Geometry check sheet. Reference: the model listing, model coordinates, mm. Face numbers are marked on the shaded views. A direction names the side the tool comes from. Coordinates: 2 decimals unless noted, no trailing zeros. Write each loop counter-clockwise with the first axis right and the second up, starting at its lowest first coordinate (ties: lowest second). Pieces come first, ordered by that corner, then holes. Notation, with made-up numbers: (88, -6) -> (139, -6) arc R19 cw to (139, 24) -> close; hole circle Ø9 at (18, -39.75). An arc over 180 degrees is marked (long way). Answer in a Markdown table with one row per item. Add a question column.
1. Cross-section at A-A on x = 19. Record the cut outline in (y, z), and give its area (3 significant figures).
2. Set-up check for the marked faces 4, 5, 6 and 7: record each of +Z, -Z, +X, -X, +Y, -Y from which the full face is reachable in a straight line by a thin tool's end or side.
3. Depth check by flat-ended pin: P1, Ø1.8, axis at x = 2, z = 2, coming from the -Y side; P2, Ø11.5, axis at x = 26, z = 24, coming from the +Y side; P3, Ø6, axis at y = 28, z = 21, coming from the -X side; P4, Ø1, axis at x = 25, y = 30, coming from the -Z side. Enter the tip coordinate at first touch or a pass-through.
4. Scan lines: L1, parallel to X at y = 1, z = 2; L2, parallel to Y at x = 3, z = 13.5; L3, parallel to Y at x = 22, z = 20.5. Record each from-to range of solid material in increasing order. Write a range as from..to.
5. Cross-section at B-B on z = 36. Record the cut outline in (x, y), and give its area (3 significant figures).
6. Cross-section at C-C on y = -1. Record the cut outline in (x, z), and give its area (3 significant figures).
7. Cross-section at D-D on z = 19. Record the cut outline in (x, y).
8. Mould release check, pull along Z, two halves, no side actions. Record for the marked faces 1, 2 and 3: pulls with the +Z half, pulls with the -Z half, needs draft (parallel to the pull), parting line crosses it, or undercut.
```python
from build123d import *

# Parameters (mm, degrees)
SKETCH_1_W      = 38
SKETCH_1_H      = 38
SKETCH_1_R      = 1
EXTRUDE_1_DEPTH = 1.5
SKETCH_2_R      = 0.636700884
SKETCH_2_R_2    = 0.447912605
SKETCH_2_R_3    = 0.577059181
SKETCH_2_R_4    = 0.454786346
EXTRUDE_2_DEPTH = 12
SKETCH_3_W      = 38
SKETCH_3_H      = 38
EXTRUDE_3_DEPTH = 1.5
SKETCH_4_R      = 7
EXTRUDE_4_DEPTH = 24
SKETCH_5_W      = 23.785325885
SKETCH_5_H      = 24.83133448
SKETCH_5_W_2    = 7.276581533
SKETCH_5_H_2    = 1.922772716
EXTRUDE_5_DEPTH = 6.6


with BuildPart() as part:
    # 草图1 → 凸台-拉伸1 (new body)
    with BuildSketch(Plane(origin=(0, 0, 0), x_dir=(1, 0, 0), z_dir=(0, 1, 0))):
        with Locations((19, -19)):
            Rectangle(SKETCH_1_W, SKETCH_1_H)
        with Locations(Location((2, -2, 0), (0, 0, 270))):
            Circle(SKETCH_1_R, mode=Mode.SUBTRACT)
        with Locations(Location((36, -2, 0), (0, 0, 270))):
            Circle(SKETCH_1_R, mode=Mode.SUBTRACT)
        with Locations(Location((36, -36, 0), (0, 0, 270))):
            Circle(SKETCH_1_R, mode=Mode.SUBTRACT)
        with Locations(Location((2, -36, 0), (0, 0, 270))):
            Circle(SKETCH_1_R, mode=Mode.SUBTRACT)
    extrude(amount=EXTRUDE_1_DEPTH)

    # 草图2 → 凸台-拉伸2 (add)
    with BuildSketch(Plane(origin=(0, 1.5, 0), x_dir=(1, 0, 0), z_dir=(0, 1, 0))):
        with Locations(Location((4.128486493, -34.030688728, 0), (0, 0, 270))):
            Circle(SKETCH_2_R)
        with Locations(Location((4.765187377, -3.05973858, 0), (0, 0, 270))):
            Circle(SKETCH_2_R_2)
        with Locations(Location((32.780026277, -2.611825975, 0), (0, 0, 270))):
            Circle(SKETCH_2_R_3)
        with Locations(Location((33.644120334, -34.030688728, 0), (0, 0, 270))):
            Circle(SKETCH_2_R_4)
    extrude(amount=EXTRUDE_2_DEPTH)

    # 草图3 → 凸台-拉伸3 (add)
    with BuildSketch(Plane(origin=(0, 13.5, 0), x_dir=(1, 0, 0), z_dir=(0, 1, 0))):
        with Locations((19, -19)):
            Rectangle(SKETCH_3_W, SKETCH_3_H)
    extrude(amount=EXTRUDE_3_DEPTH)

    # 草图4 → 凸台-拉伸4 (add)
    with BuildSketch(Plane(origin=(0, 15, 0), x_dir=(1, 0, 0), z_dir=(0, 1, 0))):
        with Locations(Location((19, -19, 0), (0, 0, 270))):
            Circle(SKETCH_4_R)
    extrude(amount=EXTRUDE_4_DEPTH)

    # 草图5 → 凸台-拉伸5 (add)
    with BuildSketch(Plane(origin=(0, 0, 0), x_dir=(-1, 0, 0), z_dir=(0, -1, 0))):
        with Locations((-19.113696587, -19.568482932)):
            Rectangle(SKETCH_5_W, SKETCH_5_H)
        with Locations((-18.818085462, -0.961386358)):
            Rectangle(SKETCH_5_W_2, SKETCH_5_H_2)
    extrude(amount=EXTRUDE_5_DEPTH)


solid = part.part
```
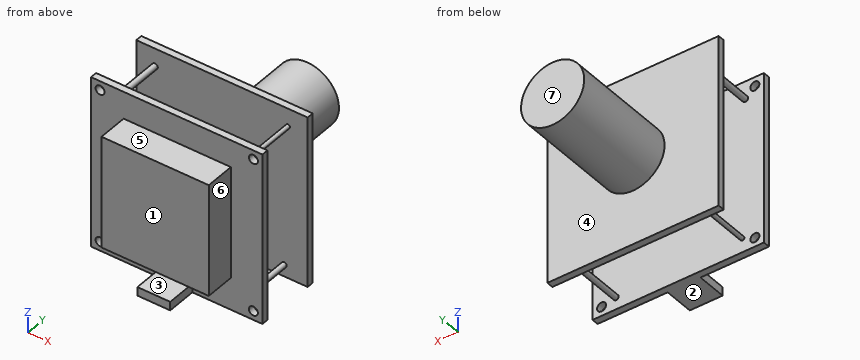
Results found:
| question | item | result |
|---|---|---|
| 1 | outline | (-6.6, 0) -> (1.5, 0) -> (1.5, 38) -> (0, 38) -> (0, 31.98) -> (-6.6, 31.98) -> (-6.6, 7.15) -> (0, 7.15) -> (0, 1.92) -> (-6.6, 1.92) -> close; (13.5, 0) -> (15, 0) -> (15, 12) -> (39, 12) -> (39, 26) -> (15, 26) -> (15, 38) -> (13.5, 38) -> close |
| 1 | area | 627 mm^2 |
| 2 | face 4 | +Y |
| 2 | face 5 | +Z, +X, -X, -Y |
| 2 | face 6 | +Z, -Z, +X, -Y |
| 2 | face 7 | +Z, -Z, +X, -X, +Y |
| 3 | P1 | stops at y = 13.5 |
| 3 | P2 | stops at y = 39 |
| 3 | P3 | stops at x = 12 |
| 3 | P4 | stops at z = 14.67 |
| 4 | L1 | x = 0..1, 3..35, 37..38 |
| 4 | L2 | y = 0..1.5, 13.5..15 |
| 4 | L3 | y = -6.6..1.5, 13.5..39 |
| 5 | outline | (0, 0) -> (1, 0) -> (1, 1.5) -> (0, 1.5) -> close; (0, 13.5) -> (38, 13.5) -> (38, 15) -> (0, 15) -> close; (3, 0) -> (35, 0) -> (35, 1.5) -> (3, 1.5) -> close; (37, 0) -> (38, 0) -> (38, 1.5) -> (37, 1.5) -> close |
| 5 | area | 108 mm^2 |
| 6 | outline | (7.22, 7.15) -> (31.01, 7.15) -> (31.01, 31.98) -> (7.22, 31.98) -> close; (15.18, 0) -> (22.46, 0) -> (22.46, 1.92) -> (15.18, 1.92) -> close |
| 6 | area | 605 mm^2 |
| 7 | outline | (0, 0) -> (7.22, 0) -> (7.22, -6.6) -> (31.01, -6.6) -> (31.01, 0) -> (38, 0) -> (38, 1.5) -> (0, 1.5) -> close; (0, 13.5) -> (38, 13.5) -> (38, 15) -> (26, 15) -> (26, 39) -> (12, 39) -> (12, 15) -> (0, 15) -> close |
| 8 | face 1 | needs draft |
| 8 | face 2 | pulls with the -Z half |
| 8 | face 3 | undercut |
